Verification items for the finished model (mm, model axes). A direction names the side the tool comes from. Round coordinates to 2 decimals unless told otherwise and drop trailing zeros. Order: outer loops, then holes, each group sorted by start corner. A loop starts at its lowest first (then second) coordinate and runs counter-clockwise, first axis right, second up. Notation, with made-up numbers: M 8,-15.5 L 23,-15.5 A23 cw 23,-1.5 Z; hole C 26,16 d5. An arc over 180 degrees is marked long. Answer as a JSON object with one key per item and string values. Group by question number.
```python
from build123d import *

# Parameters (mm, degrees)
CROQUIS1_R              = 52.5
SALIENTE_EXTRUIR1_DEPTH = 10
SALIENTE_EXTRUIR1_DRAFT = -69
CROQUIS2_R              = 78.550890647
SALIENTE_EXTRUIR2_DEPTH = 10
CROQUIS3_R              = 78.550890647
SALIENTE_EXTRUIR3_DEPTH = 10
SALIENTE_EXTRUIR3_TAPER = 69
CROQUIS4_R              = 49.5
SALIENTE_EXTRUIR4_DEPTH = 3
C_PULA1_FACE_RADIUS     = 49.5
C_PULA1_HEIGHT          = 16
CORTAR_EXTRUIR1_DEPTH   = 122.414516736
CORTAR_EXTRUIR3_REACH   = 184.352


with BuildPart() as part:
    # Croquis1 → Saliente-Extruir1 (with draft: the straight prism first)
    with BuildSketch(Plane(origin=(0, 0, 0), x_dir=(1, 0, 0), z_dir=(0, 1, 0))):
        Circle(CROQUIS1_R)
    extrude(amount=SALIENTE_EXTRUIR1_DEPTH)
    # Saliente-Extruir1: the draft: its side faces are tilted about the plane it starts from
    saliente_extruir1_sides = [part.faces().sort_by_distance(p)[0] for p in [
        (-52.5, 5, 0),
    ]]
    draft(saliente_extruir1_sides, Plane(origin=(0, 0, 0), x_dir=(1, 0, 0), z_dir=(0, 1, 0)), SALIENTE_EXTRUIR1_DRAFT)

    # Croquis2 → Saliente-Extruir2 (add)
    with BuildSketch(Plane(origin=(0, 10, 0), x_dir=(1, 0, 0), z_dir=(0, 1, 0))):
        with Locations(Location((0, 0, 0), (0, 0, 270))):
            Circle(CROQUIS2_R)
    extrude(amount=SALIENTE_EXTRUIR2_DEPTH)

    # Croquis3 → Saliente-Extruir3 (add)
    with BuildSketch(Plane(origin=(0, 20, 0), x_dir=(1, 0, 0), z_dir=(0, 1, 0))):
        with Locations(Location((0, 0, 0), (0, 0, 270))):
            Circle(CROQUIS3_R)
    extrude(amount=SALIENTE_EXTRUIR3_DEPTH, taper=SALIENTE_EXTRUIR3_TAPER)

    # Croquis4 → Saliente-Extruir4 (add)
    with BuildSketch(Plane(origin=(0, 30, 0), x_dir=(1, 0, 0), z_dir=(0, 1, 0))):
        with Locations(Location((0, 0, 0), (0, 0, 270))):
            Circle(CROQUIS4_R)
    extrude(amount=SALIENTE_EXTRUIR4_DEPTH)

    # Cúpula1: a dome of height H over a round flat face of radius A is a cap of a sphere of radius (A * A + H * H) / (2 * H)
    c_pula1_r = (C_PULA1_FACE_RADIUS * C_PULA1_FACE_RADIUS + C_PULA1_HEIGHT * C_PULA1_HEIGHT) / (2 * C_PULA1_HEIGHT)
    c_pula1_base = Plane((0, 33, 0), z_dir=(0, 1, 0))
    with Locations(c_pula1_base.offset(C_PULA1_HEIGHT - c_pula1_r)):
        c_pula1_ball = Sphere(c_pula1_r, mode=Mode.PRIVATE)
    add(split(c_pula1_ball, bisect_by=c_pula1_base, keep=Keep.TOP, mode=Mode.PRIVATE))

    # Croquis6 → Cortar-Extruir1 (cut, through all)
    with BuildSketch(Plane(origin=(0, 0, 0), x_dir=(0, 0, -1), z_dir=(1, 0, 0))):
        Polygon((-49.5, 33), (55.064393683, 0.984378507), (52.5, 0), (-52.5, 0), (-78.550890647, 10), (-78.550890647, 20), align=None)
    extrude(amount=CORTAR_EXTRUIR1_DEPTH, mode=Mode.SUBTRACT)

    # Cortar-Extruir3: up to this plane
    cortar_extruir3_end = Plane(origin=(78.550890647, 33, 49.5), z_dir=(0, -0.9561843075173418, 0.2927653839810668))
    # Croquis9 → Cortar-Extruir3 (cut, up to the surface)
    with BuildSketch(Plane.XY.offset(78.550890647), mode=Mode.PRIVATE) as cortar_extruir3_sk1:
        Polygon((0, 0), (-21.79627584, 30), (0, 30), align=None)
    cortar_extruir3_tool1 = split(extrude(cortar_extruir3_sk1.sketch, amount=-CORTAR_EXTRUIR3_REACH, mode=Mode.PRIVATE), bisect_by=cortar_extruir3_end, keep=Keep.BOTH, mode=Mode.PRIVATE)
    add(cortar_extruir3_tool1.solids().sort_by_distance((-7.265425, 20, 78.550891))[0], mode=Mode.SUBTRACT)


solid = part.part
```
Q1. Thickness scan on line 1 (X direction, y = 19.5, z = -61); line 2 (Z direction, x = 23, y = 39.5); line 3 (Z direction, x = 1.5, y = 38). Record the ranges inside material, lowest first. Write a range as from..to.
Q2. Cross-section at A-A, the plane z = 0. Record the cut outline in (x, y), then the cut area to 3 significant figures.
Q3. Gauge pin test, flat ends, axial feed: pin 1 Ø5 at (x, z) = (-10, 42.5) entering from -Y; pin 2 Ø5 at (x, z) = (-62.5, -39) entering from -Y; pin 3 Ø10 at (y, z) = (13.5, 34.5) entering from +X; pin 4 Ø2 at (y, z) = (33.5, -14) entering from -X. Record the tip position at first contact, or that the pin passes through.
Q4. Release check for a two-part mould opening along Y. For faces 1 (the face through (15.8, 30, -47.2)), 2 (the face through (-11, 30, 44)), 3 (the face through (-42.803, 0.486, -32.536)) record: released by +Y, released by -Y, zero draft, split by the parting line, or undercut.
Q5. Tool access check on faces 4 (the face through (2.18, 31.48, -49.45)), 5 (the face through (-48.238, 14.93, -61.995)). Record the directions out of +Z, -Z, +X, -X, +Y, -Y that give a thin tool (end or side, any length) a straight path to the whole face; none if there is none.
Q6. Cross-section at B-B, the plane y = 17.5. Record the cut outline in (x, z).
Q7. Cross-section at C-C, the plane y = 25.5. Record the cut outline in (x, z).
Conclusion:
{
 "1": {"line 1": "-49.49..49.49", "line 2": "-31.43..31.43", "line 3": "-41.68..41.68"},
 "2": {"outline": "M -78.55,10 L -52.5,0 L 0,0 L -12.96,17.84 L 78.55,17.84 L 78.55,20 L 52.5,30 L 49.5,30 L 49.5,33 A84.57 ccw -49.5,33 L -49.5,30 L -52.5,30 L -78.55,20 Z", "area": "4,180 mm2"},
 "3": {"pin 1": "y = 0", "pin 2": "y = 7.17", "pin 3": "x = -6.18", "pin 4": "x = -47.73"},
 "4": {"face 1": "released by +Y", "face 2": "undercut", "face 3": "released by -Y"},
 "5": {"face 4": "+Y", "face 5": "+Y, -Y"},
 "6": {"outline": "M -12.71,-1.12 L -12.71,77.52 A78.55 ccw long 78.54,-1.12 Z"},
 "7": {"outline": "M -18.53,25 L -18.53,61.49 A64.22 ccw long 59.16,25 Z"}
}
